Read the model definition and answer for the solid it produces. Units are mm, in the model's axes. Face numbers are marked on the shaded views. A direction names the side the tool comes from. Give positions to 0.01 mm unless a question says otherwise; leave off trailing zeros. Order: outer loops, then holes, each group sorted by start corner. A loop starts at its lowest first (then second) coordinate and runs counter-clockwise, first axis right, second up. Notation, with made-up numbers: (30.5, -14.5) -> (78.5, -14.5) arc R31 cw to (78.5, 11.5) -> close; hole circle Ø3 at (-36, -30). An arc over 180 degrees is marked (long way). One line per item, written item: value. Start each with the question number.
Autodesk Inventor part; units mm, degrees
ref_plane "YZ Plane" through (0, 0, 0) normal (1, 0, 0) x (0, 1, 0)
ref_plane "XZ Plane" through (0, 0, 0) normal (0, 1, 0) x (-1, 0, 0)
ref_plane "XY Plane" through (0, 0, 0) normal (0, 0, 1) x (1, 0, 0)
sketch "Sketch1" plane through (0, 0, 0) normal (0, 0, 1) x (1, 0, 0)
  line L0 (-25, 25) -> (25, 25)
  line L1 (25, 25) -> (25, -25)
  line L2 (25, -25) -> (-25, -25)
  line L3 (-25, -25) -> (-25, 25)
  line L4 (-10, 10) -> (10, 10)
  line L5 (10, 10) -> (10, -10)
  line L6 (10, -10) -> (-10, -10)
  line L7 (-10, -10) -> (-10, 10)
  point P0 (0, 0)
  dimension "d0" = 50
  dimension "d1" = 50
  dimension "d2" = 25
  dimension "d3" = 25
  dimension "d4" = 20
  dimension "d5" = 20
  dimension "d6" = 10
  dimension "d7" = 10
extrude "Extrusion1" add sketch "Sketch1" along normal mid plane 50
sketch "Sketch2" plane through (-25, -25, 25) normal (-1, 0, 0) x (0, 0, 1)
  circle A0 centre (-25, 25) radius 5
  dimension "d10" = 10
extrude "Extrusion2" add sketch "Sketch2" along normal blind 15
mirror "Mirror1" about plane through (0, 0, 0) normal (1, 0, 0) of "Extrusion2"
properties part number "prismaticFulcrum" material "Stainless Steel"
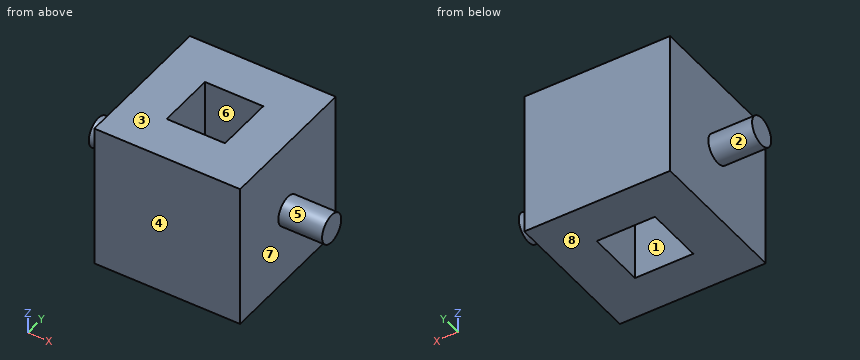
Item 1: Flat-ended cylindrical pins translate along their axes: pin 1 (10 mm diameter, centred on y = 6, z = -18, fed in from +X); pin 2 (8 mm diameter, centred on y = -1.5, z = -12, fed in from -X). Find the tip coordinate at first contact, or state that the pin passes through.
Item 2: For a pull along X with two mould halves and no side action, classify the marked faces 6, 7 and 8 as +X half, -X half, draft (parallel to the pull), parting line (faces both ways), or undercut.
Item 3: Find section C-C on z = 9.5. Write down the section's boundary in (x, y), then the cut area to 3 significant figures.
Item 4: Find section A-A on y = -8.5. Write down the section's boundary in (x, z).
Item 5: Find section D-D on y = -3. Write down the section's boundary in (x, z), then the cut area to 3 significant figures.
Item 6: Find the intervals of material crossed by line 1 (Y direction, x = 6.5, z = -18.5); line 2 (X direction, y = -1.5, z = 4.5), in increasing order. Write a range as from..to.
Item 7: A tool of negligible diameter and unlimited length cuts with its end or side. For the marked faces 1, 2, 3, 4 and 5, from which of +Z, -Z, +X, -X, +Y, -Y can it reach the whole face along a straight path? Write none if from no direction.
Checks:
1. pin 1: x = 25
1. pin 2: x = -25
2. face 6: undercut
2. face 7: +X half
2. face 8: draft
3. outline: (-25, -25) -> (25, -25) -> (25, 25) -> (-25, 25) -> close; hole (-10, -10) -> (10, -10) -> (10, 10) -> (-10, 10) -> close
3. area: 2,100 mm2
4. outline: (-25, -25) -> (-10, -25) -> (-10, 25) -> (-25, 25) -> close; (10, -25) -> (25, -25) -> (25, 25) -> (10, 25) -> close
5. outline: (-40, -4) -> (-25, -4) -> (-25, -25) -> (-10, -25) -> (-10, 25) -> (-25, 25) -> (-25, 4) -> (-40, 4) -> close; (10, -25) -> (25, -25) -> (25, -4) -> (40, -4) -> (40, 4) -> (25, 4) -> (25, 25) -> (10, 25) -> close
5. area: 1,740 mm2
6. line 1: -25..-10, 10..25
6. line 2: -40..-10, 10..40
7. face 1: +Z, -Z
7. face 2: -X
7. face 3: +Z, +X, -X, +Y, -Y
7. face 4: +Z, -Z, +X, -X, -Y
7. face 5: +X
